Design review of the part shown in the three views and the two pictorial views. Dimensions are in mm from the part's minimum x, y and z. A direction names the side the tool comes from. Round coordinates to 2 decimals unless told otherwise and drop trailing zeros. Loops run counter-clockwise (first coordinate to the right, second up) from the corner with the lowest first, then second, coordinate; pieces in that order, holes last. Notation, with made-up numbers: (46, 58) - (80, 58) arc R12 ccw to (80, 76) - close; hole circle Ø3 at (18, 89.5). An arc over 180 degrees is marked (long way). Return JSON: item names as keys, results as strings. Group by question number.
(1) We need section A-A, the plane y = 33. Write out the cut boundary in (x, z), and give its area (3 significant figures).
(2) Wall thickness on L1, parallel to Y at x = 40.5, z = 1.35; L2, parallel to Y at x = 40, z = 1; L3, parallel to Y at x = 33, z = 15.5: over which ranges is each line inside the solid? List them lowest first. Write a range as [from, to].
(3) We need section C-C, the plane z = 34. Write out the cut boundary in (x, y), and give its area (3 significant figures).
(4) We need section B-B, the plane x = 25. Write out the cut boundary in (y, z).
(5) Clearance check with flat-ended pins moving along their axes: pin 1 (1 mm diameter, centred on x = 15.5, z = 23.5, fed in from +Y); pin 2 (3.5 mm diameter, centred on x = 9.5, y = 14.5, fed in from +Z). State where each tip first meets the part, or that it passes through.
(6) For the marked faces 1 and 2, list the 3-axis set-ups (+Z, -Z, +X, -X, +Y, -Y) from which the entire face can be reached by the end or side of a thin tool; tool diameter is ignored.
(7) We need section D-D, the plane x = 40. Write out the cut boundary in (y, z).
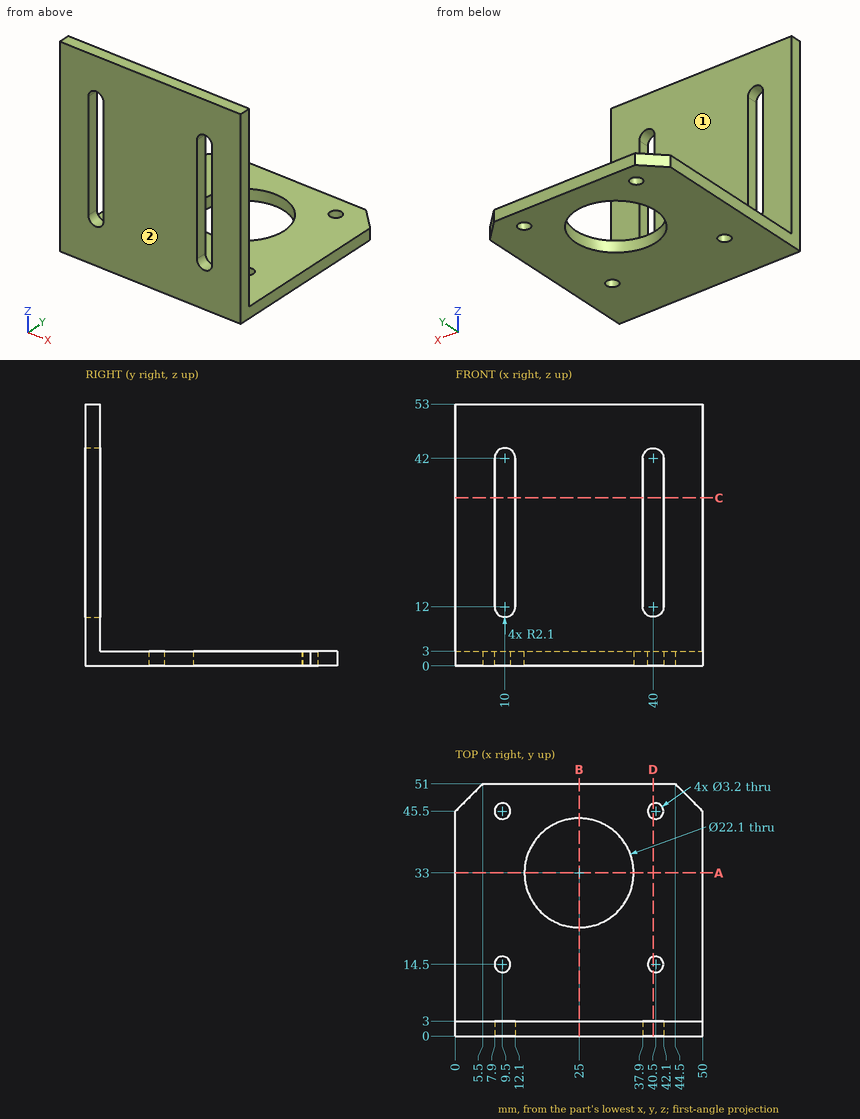
Solutions:
{
 "1": {"outline": "(0, 0) - (13.95, 0) - (13.95, 3) - (0, 3) - close; (36.05, 0) - (50, 0) - (50, 3) - (36.05, 3) - close", "area": "83.7 mm^2"},
 "2": {"L1": "[0, 12.9], [16.1, 43.9], [47.1, 51]", "L2": "[0, 12.98], [16.02, 43.98], [47.02, 51]", "L3": "[0, 3]"},
 "3": {"outline": "(0, 0) - (7.9, 0) - (7.9, 3) - (0, 3) - close; (12.1, 0) - (37.9, 0) - (37.9, 3) - (12.1, 3) - close; (42.1, 0) - (50, 0) - (50, 3) - (42.1, 3) - close", "area": "125 mm^2"},
 "4": {"outline": "(0, 0) - (21.95, 0) - (21.95, 3) - (3, 3) - (3, 53) - (0, 53) - close; (44.05, 0) - (51, 0) - (51, 3) - (44.05, 3) - close"},
 "5": {"pin 1": "y = 3", "pin 2": "z = 3"},
 "6": {"face 1": "+Z, +X, -X, +Y", "face 2": "+Z, -Z, +X, -X, -Y"},
 "7": {"outline": "(0, 0) - (12.98, 0) - (12.98, 3) - (3, 3) - (3, 9.9) - (0, 9.9) - close; (0, 44.1) - (3, 44.1) - (3, 53) - (0, 53) - close; (16.02, 0) - (43.98, 0) - (43.98, 3) - (16.02, 3) - close; (47.02, 0) - (51, 0) - (51, 3) - (47.02, 3) - close"}
}
